Can you work these out from the drawing? Everything is in mm from the part's minimum corner. A direction names the side the tool comes from. Round coordinates to 2 decimals unless told otherwise and drop trailing zeros. Loops run counter-clockwise (first coordinate to the right, second up) from the corner with the lowest first, then second, coordinate; pieces in that order, holes last. Notation, with made-up numbers: M -30.5,-35.5 L 18.5,-35.5 A9 cw 18.5,-21.5 Z; hole C -12.75,-14 d8. An arc over 180 degrees is marked long. Use a Markdown table: item, result.
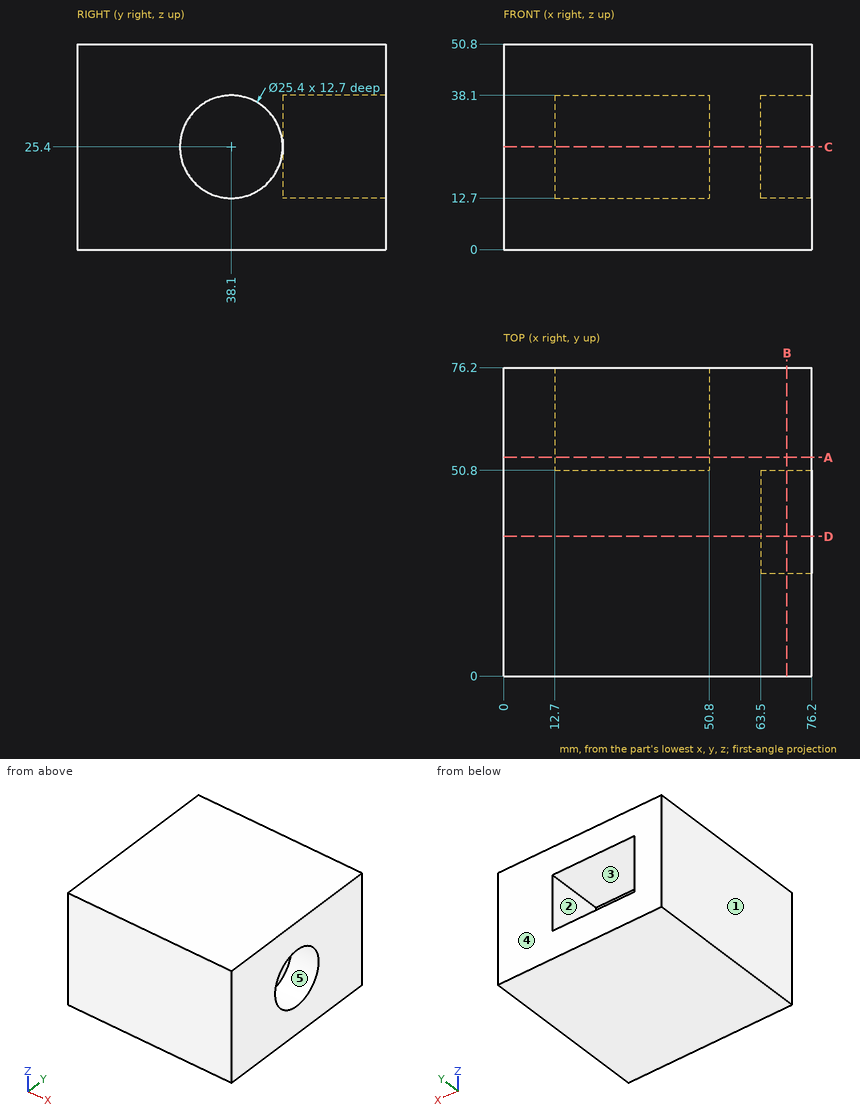
1. Imagine slicing it at A-A, the plane y = 54. Write out the boundary of the cut face in (x, z), then the cut area to 3 significant figures.
Answer sheet:
| item | result |
|---|---|
| outline | M 0,0 L 76.2,0 L 76.2,50.8 L 0,50.8 Z; hole M 12.7,12.7 L 50.8,12.7 L 50.8,38.1 L 12.7,38.1 Z |
| area | 2,900 mm2 |
2. We'd pull the mould along Y, two halves only. Please class the marked faces 3, 4 and 5: +Y half, -Y half, draft (parallel to the pull), parting line (faces both ways), or undercut.
Answer sheet:
| item | result |
|---|---|
| face 3 | draft |
| face 4 | +Y half |
| face 5 | undercut |
3. Imagine slicing it at D-D, the plane y = 34.5. Write out the boundary of the cut face in (x, z).
Answer sheet:
| item | result |
|---|---|
| outline | M 0,0 L 76.2,0 L 76.2,13.22 L 63.5,13.22 L 63.5,37.58 L 76.2,37.58 L 76.2,50.8 L 0,50.8 Z |
4. For pin 1 Ø12 at (y, z) = (11.5, 8.5) entering from -X; pin 2 Ø7.5 at (x, z) = (37.5, 28.5) entering from +Y, each with a flat end and sliding along its axis, tell me the tip position at first contact or that it passes through.
Answer sheet:
| item | result |
|---|---|
| pin 1 | x = 0 |
| pin 2 | y = 50.8 |
5. Imagine slicing it at B-B, the plane x = 70. Write out the boundary of the cut face in (y, z), then the cut area to 3 significant figures.
Answer sheet:
| item | result |
|---|---|
| outline | M 0,0 L 76.2,0 L 76.2,50.8 L 0,50.8 Z; hole C 38.1,25.4 d25.4 |
| area | 3,360 mm2 |
6. I need wall thicknesses on probe 1 along Y at (x, z) = (71, 25.4); probe 2 along X at (y, z) = (58.5, 13); probe 3 along Z at (x, y) = (33, 52.5). Which ranges of each line are inside material? Lowest first, please. Write a range as from..to.
Answer sheet:
| item | result |
|---|---|
| probe 1 | 0..25.4, 50.8..76.2 |
| probe 2 | 0..12.7, 50.8..76.2 |
| probe 3 | 0..12.7, 38.1..50.8 |
7. Imagine slicing it at C-C, the plane z = 25.4. Write out the boundary of the cut face in (x, y).
Answer sheet:
| item | result |
|---|---|
| outline | M 0,0 L 76.2,0 L 76.2,25.4 L 63.5,25.4 L 63.5,50.8 L 76.2,50.8 L 76.2,76.2 L 50.8,76.2 L 50.8,50.8 L 12.7,50.8 L 12.7,76.2 L 0,76.2 Z |
8. Which directions (+Z, -Z, +X, -X, +Y, -Y) give clear straight access to the entire face, cutting with the end or side of a thin tool? Please do the marked faces 1 and 2.
Answer sheet:
| item | result |
|---|---|
| face 1 | +Z, -Z, -X, +Y, -Y |
| face 2 | +Y |
